Geometry: final body of the model. Coordinates: model frame, mm. Coordinates: 2 decimals unless noted, no trailing zeros. Order: outer loops, then holes, each group sorted by start corner. A loop starts at its lowest first (then second) coordinate and runs counter-clockwise, first axis right, second up. Notation, with made-up numbers: M -37,-18 L 3,-18 A17 ccw 3,8 Z; hole C -36.5,-9 d3. An arc over 180 degrees is marked long. Write item = value, one per line.
from build123d import *

# Parameters (mm, degrees)
F0_W     = 19.783596
F0_H     = 19.73808
F1_DEPTH = 63.5
F2_SIZE  = 9.779
F3_SIZE  = 7.62


with BuildPart() as f1:
    # F0 (on Top) → F1 (new body)
    with BuildSketch(Plane.XY):
        with Locations((-9.891798, 9.86904)):
            Rectangle(F0_W, F0_H)
    extrude(amount=F1_DEPTH)

    # F2
    f2_edges = [f1.edges().sort_by_distance(p)[0] for p in [
        (-9.891798, 0, 63.5),
        (0, 9.86904, 63.5),
        (-9.891798, 19.73808, 63.5),
        (-19.783596, 9.86904, 63.5),
    ]]
    chamfer(f2_edges, length=F2_SIZE)

    # F3
    f3_edges = [f1.edges().sort_by_distance(p)[0] for p in [
        (-9.891798, 0, 0),
        (0, 9.86904, 0),
        (-9.891798, 19.73808, 0),
        (-19.783596, 9.86904, 0),
    ]]
    chamfer(f3_edges, length=F3_SIZE)


solid = f1.part
1) Section B-B, the plane x = -4.5. Return loops of the section in (y, z), and give its area (3 significant figures).
Numbers:
outline = M 0,7.62 L 4.5,3.12 L 15.24,3.12 L 19.74,7.62 L 19.74,53.72 L 15.24,58.22 L 4.5,58.22 L 0,53.72 Z
area = 1,050 mm²
2) Line query: L1, parallel to Z at x = -1.25, y = 12.75; L2, parallel to Z at x = -17, y = 13.25; L3, parallel to Y at x = -11, z = 57.5. Output: solid intervals per line, ascending.
Numbers:
L1 = 6.37 to 54.97
L2 = 4.84 to 56.5
L3 = 3.78 to 15.96
3) Section C-C, the plane z = 58.5. Return loops of the section in (x, y).
Numbers:
outline = M -15,4.78 L -4.78,4.78 L -4.78,14.96 L -15,14.96 Z
4) Pin query (flat end, axial travel): pin 1 (1.5 mm diameter, centred on x = -16, y = 3, fed in from -Z); pin 2 (8 mm diameter, centred on x = -3, y = 4, fed in from +Z). Return the tip coordinate at first contact, or that it passes through.
Numbers:
pin_1 = 3.87
pin_2 = 60
5) Section A-A, the plane y = 6. Return loops of the section in (x, z).
Numbers:
outline = M -19.78,7.62 L -13.78,1.62 L -6,1.62 L 0,7.62 L 0,53.72 L -6,59.72 L -13.78,59.72 L -19.78,53.72 Z
